The listing builds one solid part. Answer for the finished solid, in the listing's coordinates (mm). A direction names the side the tool comes from. Coordinates: 2 decimals unless noted, no trailing zeros. Write each loop counter-clockwise with the first axis right and the second up, starting at its lowest first coordinate (ties: lowest second). Pieces come first, ordered by that corner, then holes. Notation, with made-up numbers: M -4,40.5 L 11,40.5 A19 cw 11,72.5 Z; hole C 59,24.25 d2. An arc over 180 degrees is marked long. Answer as a JSON object with one key per item and string values. Group by question number.
from build123d import *

# Parameters (mm, degrees)
SKETCH_W        = 11.75
SKETCH_H        = 32.3
PAD_DEPTH       = 22.5
SKETCH001_W     = 4.875
SKETCH001_H     = 15.6
SKETCH001_H_2   = 4.4
POCKET_DEPTH    = 11.751
PAD001_DEPTH    = 4.1
SKETCH003_R     = 2.43
PAD002_DEPTH    = 2.15
SKETCH004_R     = 1.05
POCKET001_DEPTH = 5


with BuildPart() as part:
    # Sketch → Pad (new body)
    with BuildSketch(Plane.XZ):
        with Locations((5.875, 16.15)):
            Rectangle(SKETCH_W, SKETCH_H)
    extrude(amount=PAD_DEPTH)

    # Sketch001 (on Face2 of Pad) → Pocket (cut, through all)
    with BuildSketch(Plane(origin=(11.75, 0, 0), x_dir=(0, 0, 1), z_dir=(1, 0, 0))):
        with Locations((29.8625, 7.8)):
            Rectangle(SKETCH001_W, SKETCH001_H)
        with Locations((29.8625, 20.3)):
            Rectangle(SKETCH001_W, SKETCH001_H_2)
        with Locations((2.4375, 20.3)):
            Rectangle(SKETCH001_W, SKETCH001_H_2)
        with Locations((2.4375, 7.8)):
            Rectangle(SKETCH001_W, SKETCH001_H)
    extrude(amount=-POCKET_DEPTH, mode=Mode.SUBTRACT)

    # Sketch002 (on Face13 of Pocket) → Pad001 (join)
    with BuildSketch(Plane.XZ.offset(22.5)):
        with BuildLine():
            ThreePointArc((8.8125, 16.462101), (5.875, 27.425), (2.9375, 16.462101))
            ThreePointArc((2.9375, 16.462101), (5.875, 13.524601), (8.8125, 16.462101))
        make_face()
    extrude(amount=PAD001_DEPTH)

    # Sketch003 (on Face19 of Pad001) → Pad002 (join)
    with BuildSketch(Plane.XZ.offset(26.6)):
        with Locations((5.875, 21.55)):
            Circle(SKETCH003_R)
    extrude(amount=PAD002_DEPTH)

    # Sketch004 (on Face4 of Pad002) → Pocket001 (cut)
    with BuildSketch(Plane.XZ.offset(18.1)):
        with Locations((5.875, 29.925)):
            Circle(SKETCH004_R)
        with Locations((5.875, 2.375)):
            Circle(SKETCH004_R)
    extrude(amount=-POCKET001_DEPTH, mode=Mode.SUBTRACT)


solid = part.part
Item 1: For a pull along Z with two mould halves and no side action, classify faces 5 (the face through (6, 0, 16)), 6 (the face through (4.826, -16.868, 2.421)), 7 (the face through (6.996, -27.66, 19.394)) as +Z half, -Z half, draft (parallel to the pull), parting line (faces both ways), or undercut.
Item 2: A tool of negligible diameter and unlimited length cuts with its end or side. For faces 1 (the face through (10, -22.5, 26)), 2 (the face through (6, -20, 27.425)), 3 (the face through (6, -18.1, 1)), 4 (the face through (6, -8, 4.875)), from which of +Z, -Z, +X, -X, +Y, -Y can it reach the whole face along a straight path? Write none if from no direction.
Item 3: A cutting plane is placed at B-B, the plane z = 15. Write down the section's boundary in (x, y).
Item 4: Flat-ended cylindrical pins translate along their axes: pin 1 Ø1 at (x, z) = (6.5, 27) entering from -Y; pin 2 Ø4 at (x, z) = (5.5, 2.5) entering from +Y; pin 3 Ø4 at (x, z) = (4.5, 3) entering from -Y. Find the tip coordinate at first contact, or state that the pin passes through.
Item 5: A cutting plane is placed at C-C, the plane y = -16.5. Write down the section's boundary in (x, z) (3 decimals), and give its area (3 significant figures).
Item 6: A cutting plane is placed at A-A, the plane x = 1.25. Write down the section's boundary in (y, z) (3 decimals).
Item 7: Consider L1, parallel to Z at x = 9, y = -20.75 (3 decimals); L2, parallel to Y at x = 10.25, z = 2; L3, parallel to Y at x = 5.75, z = 16.5. Determine where each line is inside the solid, lowest interval first. Write a range as from..to.
Answer:
{
 "1": {"face 5": "draft", "face 6": "undercut", "face 7": "parting line"},
 "2": {"face 1": "+Z, +X, -Y", "face 2": "+Z, +X, -X, -Y", "face 3": "-Z, +X, -X, -Y", "face 4": "-Z, +X, -X, +Y"},
 "3": {"outline": "M 0,-22.5 L 3.33,-22.5 L 3.33,-26.6 L 8.42,-26.6 L 8.42,-22.5 L 11.75,-22.5 L 11.75,0 L 0,0 Z"},
 "4": {"pin 1": "y = -26.6", "pin 2": "y = -15.6", "pin 3": "y = -22.5"},
 "5": {"outline": "M 0,0 L 11.75,0 L 11.75,32.3 L 0,32.3 Z; hole C 5.875,2.375 d2.1; hole C 5.875,29.925 d2.1", "area": "373 mm2"},
 "6": {"outline": "M -26.6,17.927 L -22.5,17.927 L -22.5,4.875 L -18.1,4.875 L -18.1,0 L -15.6,0 L -15.6,4.875 L 0,4.875 L 0,27.425 L -15.6,27.425 L -15.6,32.3 L -18.1,32.3 L -18.1,27.425 L -22.5,27.425 L -22.5,25.173 L -26.6,25.173 Z"},
 "7": {"L1": "4.875..27.425", "L2": "-18.1..-15.6", "L3": "-26.6..0"}
}
